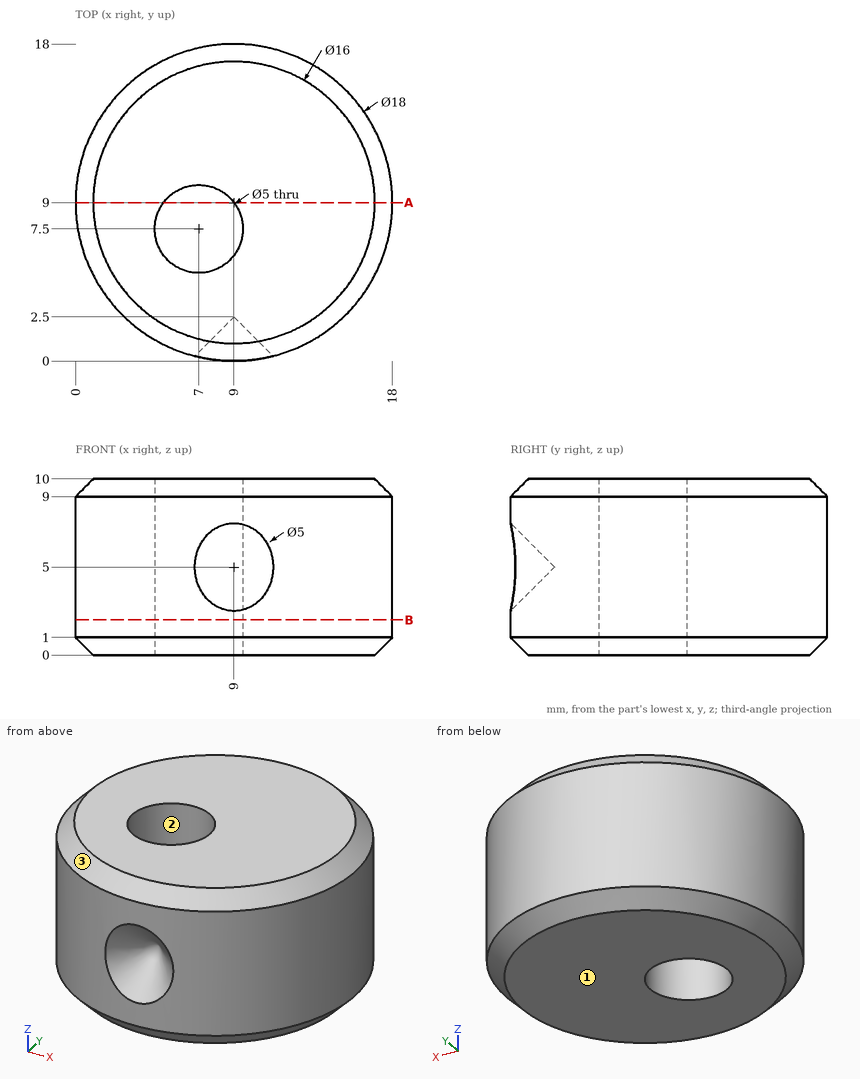
Input: dimensioned drawing with shaded views. Units: mm. Origin: part minimum x, y, z. Round coordinates to 2 decimals unless told otherwise and drop trailing zeros. Loops run counter-clockwise (first coordinate to the right, second up) from the corner with the lowest first, then second, coordinate; pieces in that order, holes last. Notation, with made-up numbers: (76, 78.5) -> (120, 78.5) arc R10 ccw to (120, 95.5) -> close; hole circle Ø8 at (79, -37). An arc over 180 degrees is marked (long way). Answer as a JSON object with one key per item and string values. Group by question number.
1) Section query B-B on z = 2. Output: boundary loops of the cut face in (x, y).
2) Ray query, L1, parallel to Y at x = 7.25, z = 5.75; L2, parallel to Y at x = 7, z = 5; L3, parallel to Y at x = 9.75, z = 8.25. Return the intervals inside material, ascending.
3) Pin query (flat end, axial travel): pin 1 (1.5 mm diameter, centred on y = 2, z = 8.5, fed in from -X); pin 2 (1 mm diameter, centred on x = 7.5, y = 9, fed in from -Z) (3 decimals); pin 3 (3 mm diameter, centred on x = 3.5, z = 1.5, fed in from +Y); pin 4 (2 mm diameter, centred on y = 15.5, z = 4, fed in from +X). Return the tip coordinate at first contact, or that it passes through.
4) Draft query along X for the marked faces 1, 2 and 3. Return one class per face: +X half, -X half, draft (parallel to the pull), parting line (faces both ways), or undercut.
5) Section query A-A on y = 9. Output: boundary loops of the cut face in (x, z), plus the area to 3 significant figures.
Reply:
{
 "1": {"outline": "circle Ø18 at (9, 9); hole circle Ø5 at (7, 7.5)"},
 "2": {"L1": "y = 0.6 to 5.01, 9.99 to 17.83", "L2": "y = 0.5 to 5, 10 to 17.77", "L3": "y = 0.03 to 17.97"},
 "3": {"pin 1": "stops at x = 2.52", "pin 2": "passes through", "pin 3": "stops at y = 17.06", "pin 4": "stops at x = 16.12"},
 "4": {"face 1": "draft", "face 2": "undercut", "face 3": "parting line"},
 "5": {"outline": "(0, 1) -> (1, 0) -> (5, 0) -> (5, 10) -> (1, 10) -> (0, 9) -> close; (9, 0) -> (17, 0) -> (18, 1) -> (18, 9) -> (17, 10) -> (9, 10) -> close", "area": "138 mm2"}
}
